Job drawing, mm, ordinate dimensions from the low corner. One solid piece. A direction names the side the tool comes from. Coordinates: 2 decimals unless noted, no trailing zeros. Order: outer loops, then holes, each group sorted by start corner. A loop starts at its lowest first (then second) coordinate and runs counter-clockwise, first axis right, second up. Notation, with made-up numbers: M -3,24 L 5,24 A20 cw 5,32 Z; hole C 33,-24 d11. An arc over 180 degrees is marked long. Write item = value, one per line.
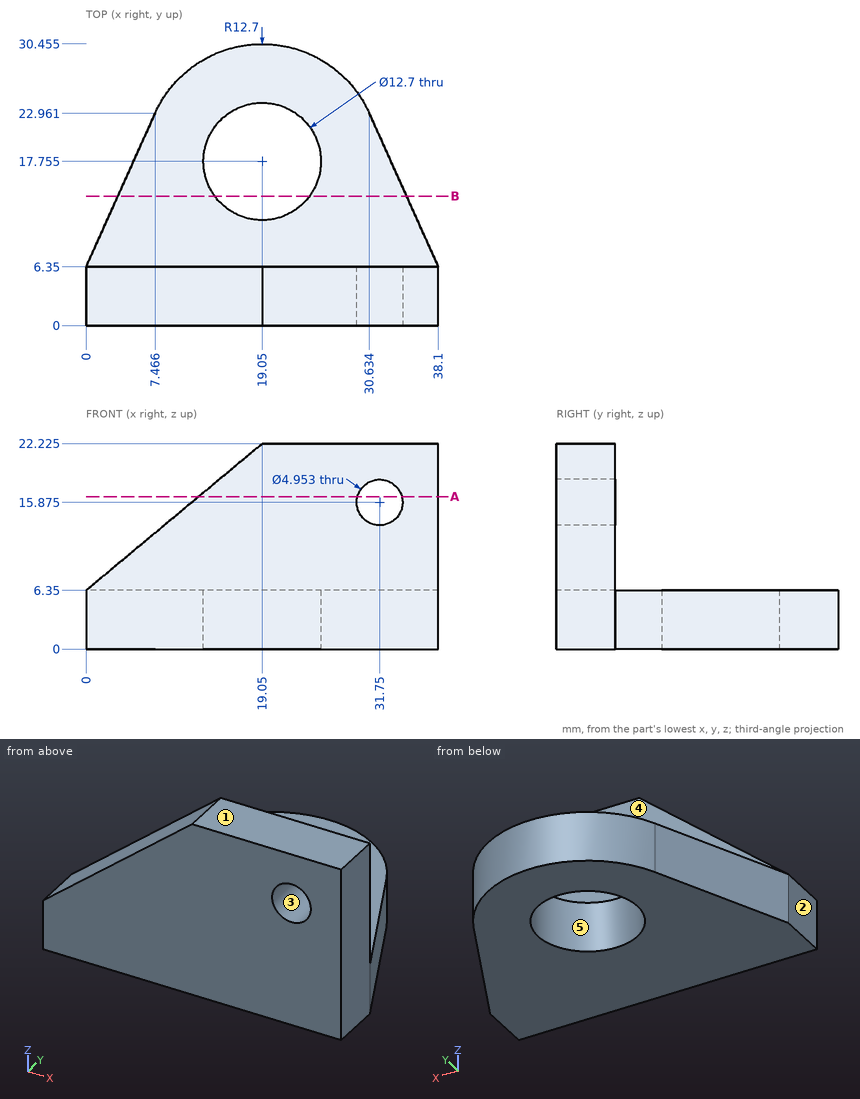
(1) Pin check, flat tips, straight feed: pin 1 Ø8 at (x, y) = (15.5, 19) entering from +Z; pin 2 Ø5 at (x, z) = (22, 14.5) entering from +Y. Stop position of each tip, or through.
Evaluation:
pin_1 = 6.35
pin_2 = 6.35
(2) Tool access for the marked faces 4 and 5: list every direction of +Z, -Z, +X, -X, +Y, -Y with a clear straight run to the whole face (end or side of a thin tool).
Evaluation:
face_4 = +Z, +X, -X, +Y
face_5 = +Z, -Z
(3) Pull direction X, two halves, no side cores. Call the marked faces 1, 2 and 3: +X half, -X half, draft (parallel to the pull), parting line (faces both ways), or undercut.
Evaluation:
face_1 = draft
face_2 = -X half
face_3 = undercut
(4) Slice it at A-A, the plane z = 16.5. Write the cut outline in (x, y), then the cut area to 3 significant figures.
Evaluation:
outline = M 12.18,0 L 29.35,0 L 29.35,6.35 L 12.18,6.35 Z; M 34.15,0 L 38.1,0 L 38.1,6.35 L 34.15,6.35 Z
area = 134 mm²
(5) Wall check: line 1 (Y direction, x = 19.05, z = 1.5) (1 decimal); line 2 (Z direction, x = 31.75, y = 3.5) (1 decimal); line 3 (Y direction, x = 17, z = 11). Give the ranges that are in metal, low to high. Write a range as from..to.
Evaluation:
line_1 = 0..11.4, 24.1..30.5
line_2 = 0..13.4, 18.4..22.2
line_3 = 0..6.35
(6) Slice it at B-B, the plane y = 14. Write the cut outline in (x, z).
Evaluation:
outline = M 3.44,0 L 13.93,0 L 13.93,6.35 L 3.44,6.35 Z; M 24.17,0 L 34.66,0 L 34.66,6.35 L 24.17,6.35 Z
